from build123d import *

# Parameters (mm, degrees)
SKETCH1_W           = 6.4
SKETCH1_H           = 6.4
BOSS_EXTRUDE1_DEPTH = 1.3
SKETCH2_W           = 0.8
SKETCH2_H           = 6.4
BOSS_EXTRUDE2_DEPTH = 0.0001
SKETCH3_W           = 0.8
SKETCH3_H           = 1.22
SKETCH3_H_2         = 1.016
BOSS_EXTRUDE3_DEPTH = 3.2
CHAMFER1_SIZE       = 0.254
SKETCH4_R           = 0.24
BOSS_EXTRUDE4_DEPTH = 3.2001
FILLET1_R           = 0.125
SKETCH5_R           = 2.4
SKETCH5_R_2         = 2.0825
SKETCH5_R_3         = 0.381
BOSS_EXTRUDE5_DEPTH = 4.1
CUT_EXTRUDE1_START  = -1.524
SKETCH7_R           = 0.381
CUT_EXTRUDE1_DEPTH  = 1.524
SKETCH8_R           = 0.381
BOSS_EXTRUDE6_DEPTH = 0.762
BOSS_EXTRUDE6_TAPER = 15
FILLET2_R           = 0.127
FILLET3_R           = 0.127


with BuildPart() as part:
    # Sketch1 → Boss-Extrude1 (new body)
    with BuildSketch(Plane(origin=(0, 0, 0), x_dir=(1, 0, 0), z_dir=(0, 1, 0))):
        Rectangle(SKETCH1_W, SKETCH1_H)
    extrude(amount=BOSS_EXTRUDE1_DEPTH)

    # Sketch2 → Boss-Extrude2 (add)
    with BuildSketch(Plane(origin=(0, 1.3, 0), x_dir=(1, 0, 0), z_dir=(0, 1, 0))):
        with Locations((-2.8, 0)):
            Rectangle(SKETCH2_W, SKETCH2_H)
        with Locations((2.8, 0)):
            Rectangle(SKETCH2_W, SKETCH2_H)
    extrude(amount=BOSS_EXTRUDE2_DEPTH)

    # Sketch3 → Boss-Extrude3 (add)
    with BuildSketch(Plane(origin=(0, 1.3001, 0), x_dir=(1, 0, 0), z_dir=(0, 1, 0))):
        with Locations((-2.8, -2.59)):
            Rectangle(SKETCH3_W, SKETCH3_H)
        with Locations((-2.8, 0.2552)):
            Rectangle(SKETCH3_W, SKETCH3_H_2)
        with Locations((2.8, 0.2552)):
            Rectangle(SKETCH3_W, SKETCH3_H_2)
        with Locations((2.8, -2.59)):
            Rectangle(SKETCH3_W, SKETCH3_H)
    extrude(amount=BOSS_EXTRUDE3_DEPTH)

    # Chamfer1
    chamfer1_edges = [part.edges().sort_by_distance(p)[0] for p in [
        (-2.8, 4.5001, 1.98),
        (-2.8, 4.5001, 0.2528),
        (2.8, 4.5001, 0.2528),
        (2.8, 4.5001, 1.98),
    ]]
    chamfer(chamfer1_edges, length=CHAMFER1_SIZE)

    # Sketch4 → Boss-Extrude4 (add)
    with BuildSketch(Plane(origin=(0, 1.3, 0), x_dir=(1, 0, 0), z_dir=(0, 1, 0))):
        with Locations(Location((0, 0, 0), (0, 0, 90))):
            Circle(SKETCH4_R)
    extrude(amount=BOSS_EXTRUDE4_DEPTH)

    # Fillet1
    fillet1_edges = [part.edges().sort_by_distance(p)[0] for p in [
        (0, 4.5001, 0.24),
    ]]
    fillet(fillet1_edges, radius=FILLET1_R)

    # Sketch5 → Boss-Extrude5 (add)
    # profile 1 of 2: a face of its own
    with BuildSketch(Plane.XZ):
        with Locations(Location((0, 0, 0), (0, 0, 270))):
            Circle(SKETCH5_R)
        with Locations(Location((0, 0, 0), (0, 0, 270))):
            Circle(SKETCH5_R_2, mode=Mode.SUBTRACT)
    # profile 2 of 2: a face of its own
    with BuildSketch(Plane.XZ):
        with Locations(Location((0, 0, 0), (0, 0, 270))):
            Circle(SKETCH5_R_3)
    extrude(amount=BOSS_EXTRUDE5_DEPTH)

    # Sketch7 → Cut-Extrude1 (cut)
    with BuildSketch(Plane.XZ.offset(4.1).offset(CUT_EXTRUDE1_START)):
        with Locations(Location((0, 0, 0), (0, 0, 270))):
            Circle(SKETCH7_R)
    extrude(amount=CUT_EXTRUDE1_DEPTH, mode=Mode.SUBTRACT)

    # Sketch8 → Boss-Extrude6 (add)
    with BuildSketch(Plane.XZ.offset(2.576)):
        with Locations(Location((0, 0, 0), (0, 0, 270))):
            Circle(SKETCH8_R)
    extrude(amount=BOSS_EXTRUDE6_DEPTH, taper=BOSS_EXTRUDE6_TAPER)

    # Fillet2
    fillet2_edges = [part.edges().sort_by_distance(p)[0] for p in [
        (0, -3.338, 0.176822715),
    ]]
    fillet(fillet2_edges, radius=FILLET2_R)

    # Fillet3
    fillet3_edges = [part.edges().sort_by_distance(p)[0] for p in [
        (0, -4.1, 2.4),
    ]]
    fillet(fillet3_edges, radius=FILLET3_R)


solid = part.part
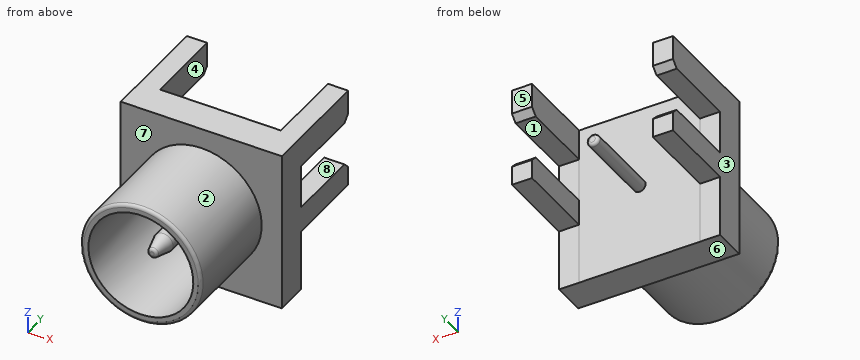
Work out the finished part from the listing and answer in its coordinate system (mm). Face numbers are marked on the shaded views. A direction names the side the tool comes from. Give positions to 0.01 mm unless a question says otherwise; leave off trailing zeros. Write each loop counter-clockwise with the first axis right and the second up, starting at its lowest first coordinate (ties: lowest second). Pieces come first, ordered by that corner, then holes.
Q1. A tool of negligible diameter and unlimited length cuts with its end or side. For the marked faces 1, 2, 3, 4 and 5, from which of +Z, -Z, +X, -X, +Y, -Y can it reach the whole face along a straight path? Write none if from no direction.
Answer:
face 1: +X, -X, +Y
face 2: -Y
face 3: +Z, -Z, -X, +Y, -Y
face 4: +Z, -Z, +Y
face 5: +Z, -Z, +X, -X, +Y
Q2. For a pull along Z with two mould halves and no side action, classify the marked faces 6, 7 and 8 as released by +Z, released by -Z, zero draft, split by the parting line, or undercut.
Answer:
face 6: released by -Z
face 7: zero draft
face 8: undercut
Q3. Straight lines are drawn through the part: L1, parallel to X at y = -1.3, z = 0; L2, parallel to X at y = -3.2, z = 0; L3, parallel to Y at x = -2, z = 2.75. For each, find the intervals that lie inside material, in ascending order.
Answer:
L1: x = -2.4 to -2.08, -0.38 to 0.38, 2.08 to 2.4
L2: x = -2.4 to -2.08, -0.21 to 0.21, 2.08 to 2.4
L3: y = 0 to 1.3
Q4. Given pin 1 (0.9 mm diameter, centred on x = 3, y = 2.5, fed in from -Z); pin 2 (1.5 mm diameter, centred on x = 2, y = -2, fed in from -Z); pin 3 (1 mm diameter, centred on x = 0, z = -1, fed in from +Y); pin 4 (1 mm diameter, centred on y = 2, z = -1.5, fed in from -X), each flat-ended and moving along its own axis, determine where each tip first touches the part or whether it passes through.
Answer:
pin 1: stops at z = -0.76
pin 2: stops at z = -2.05
pin 3: stops at y = 1.3
pin 4: passes through
Q5. The part is cut by section D-D on y = -0.75. Give the vertices of the cut face in (x, z) (1 decimal), and give its area (3 significant figures).
Answer:
outline: circle Ø4.8 at (0, 0); circle Ø0.8 at (0, 0); hole circle Ø4.2 at (0, 0)
area: 4.93 mm2
Q6. The part is cut by section B-B on x = 2.5. Give the vertices of the cut face in (y, z), and give its area (3 significant figures).
Answer:
outline: (0, -3.2) - (1.3, -3.2) - (1.3, -0.76) - (4.5, -0.76) - (4.5, 0) - (4.25, 0.25) - (1.3, 0.25) - (1.3, 1.98) - (4.25, 1.98) - (4.5, 2.23) - (4.5, 3.2) - (0, 3.2) - close
area: 15.4 mm2
Q7. The part is cut by section A-A on y = 2.25. Give the vertices of the cut face in (x, z), and give its area (3 significant figures).
Answer:
outline: (-3.2, -0.76) - (-2.4, -0.76) - (-2.4, 0.25) - (-3.2, 0.25) - close; (-3.2, 1.98) - (-2.4, 1.98) - (-2.4, 3.2) - (-3.2, 3.2) - close; circle Ø0.48 at (0, 0); (2.4, -0.76) - (3.2, -0.76) - (3.2, 0.25) - (2.4, 0.25) - close; (2.4, 1.98) - (3.2, 1.98) - (3.2, 3.2) - (2.4, 3.2) - close
area: 3.76 mm2
